Here's the drawing with two shaded views (mm, measured from the low corner). I have some questions. A direction names the side the tool comes from. Give positions to 0.01 mm unless a question says otherwise; leave off trailing zeros. Loops run counter-clockwise (first coordinate to the right, second up) from the corner with the lowest first, then second, coordinate; pieces in that order, holes last. Notation, with made-up numbers: (18, 70) -> (57, 70) arc R13 cw to (57, 77) -> close; hole circle Ø1 at (53, 46.5). An arc over 180 degrees is marked (long way). Answer in a Markdown table with one row per item. Add a question column.
Item 1: If I drill on line 1 (Y direction, x = 51.5, z = 19.05) (1 decimal); line 2 (Z direction, x = 59, y = 5.25); line 3 (Z direction, x = 37, y = 9), over which ranges is the centre line in solid material (lowest first)?
Item 2: For P1, Ø3, axis at y = 3, z = 10, coming from the +X side; P2, Ø1.5, axis at x = 46.5, y = 2.5, coming from the -Z side; P3, Ø3, axis at y = 5, z = 19.5, coming from the +X side, each with a flat end and sliding along its axis, tell me the tip position at first contact or that it passes through.
Item 3: If we section it at A-A (y = 6.35): Give the number of separate pieces and of enclosed holes in the cut face, then the cut area to 3 significant figures.
Item 4: We'd pull the mould along X, two halves only. Please class the marked faces 1, 2 and 3: released by +X, released by -X, zero draft, split by the parting line, or undercut.
Item 5: If we section it at C-C (z = 38.1): Write out the boundary of the cut face in (x, y).
Item 6: If we section it at D-D (y = 11.25): Write out the boundary of the cut face in (x, z).
Item 7: Which directions (+Z, -Z, +X, -X, +Y, -Y) give clear straight access to the entire face, cutting with the end or side of a thin tool? Please do the marked faces 4 and 5.
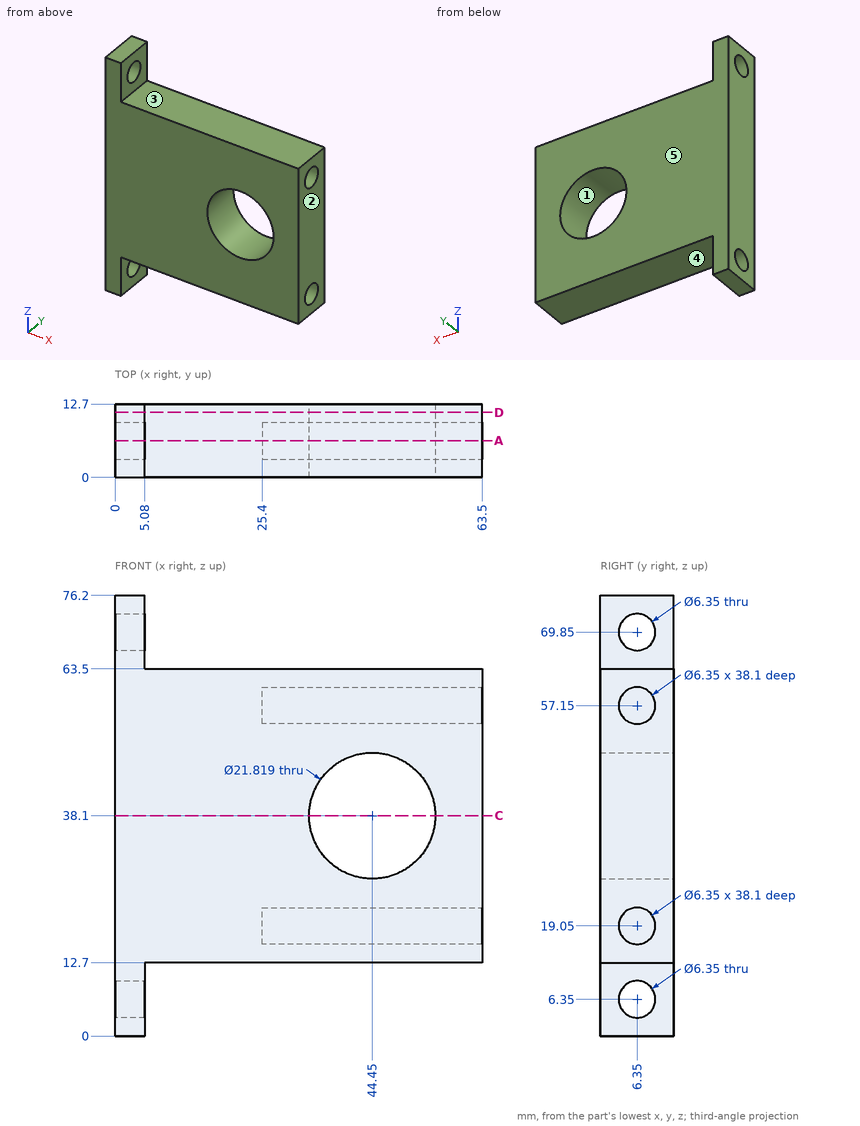
Recorded:
| question | item | result |
|---|---|---|
| 1 | line 1 | y = 0 to 3.2, 9.5 to 12.7 |
| 1 | line 2 | z = 12.7 to 16.07, 22.03 to 54.17, 60.13 to 63.5 |
| 1 | line 3 | z = 12.7 to 17.3, 20.8 to 30.13, 46.07 to 55.4, 58.9 to 63.5 |
| 2 | P1 | stops at x = 5.08 |
| 2 | P2 | stops at z = 12.7 |
| 2 | P3 | stops at x = 25.4 |
| 3 | separate pieces | 3 |
| 3 | enclosed holes | 1 |
| 3 | area | 2,430 mm^2 |
| 4 | face 1 | undercut |
| 4 | face 2 | released by +X |
| 4 | face 3 | zero draft |
| 5 | outline | (0, 0) -> (33.54, 0) -> (33.54, 12.7) -> (0, 12.7) -> close; (55.36, 0) -> (63.5, 0) -> (63.5, 12.7) -> (55.36, 12.7) -> close |
| 6 | outline | (0, 0) -> (5.08, 0) -> (5.08, 12.7) -> (63.5, 12.7) -> (63.5, 63.5) -> (5.08, 63.5) -> (5.08, 76.2) -> (0, 76.2) -> close; hole circle Ø21.82 at (44.45, 38.1) |
| 7 | face 4 | -Z, +X, +Y, -Y |
| 7 | face 5 | +Z, -Z, +X, -X, +Y |
